Can you work these out from the model? Positions are in its coordinate system, mm. A direction names the side the tool comes from. Coordinates: 2 decimals unless noted, no trailing zeros. Order: outer loops, then holes, each group sorted by start corner. A loop starts at its lowest first (then second) coordinate and runs counter-clockwise, first axis right, second up. Notation, with made-up numbers: (-24, 58) -> (15, 58) arc R32 ccw to (15, 92) -> close; hole circle Ø4 at (54.5, 8.25). An arc over 180 degrees is marked (long way). Answer as CSV lines item,"result".
from build123d import *

# Parameters (mm, degrees)
F0_W     = 101.152622
F0_H     = 124.431356
F1_DEPTH = 2
F2_W     = 101.152622
F2_H     = 124.431356
F2_W_2   = 92.701234
F2_H_2   = 115.979962
F3_DEPTH = 50
F4_W     = 165.897682
F4_H     = 37.940726
F5_DEPTH = 12


with BuildPart() as f1:
    # F0 (on Top) → F1 (new body)
    with BuildSketch(Plane.XY):
        Rectangle(F0_W, F0_H)
    extrude(amount=F1_DEPTH)

    # F2 (on face) → F3 (join)
    with BuildSketch(Plane.XY.offset(2)):
        Rectangle(F2_W, F2_H)
        Rectangle(F2_W_2, F2_H_2, mode=Mode.SUBTRACT)
    extrude(amount=F3_DEPTH)

    # F4 (on Top) → F5 (join)
    with BuildSketch(Plane.XY):
        with Locations((-26.223734, 12.385411)):
            Rectangle(F4_W, F4_H)
    extrude(amount=F5_DEPTH)


solid = f1.part
Q1. Imagine slicing it at C-C (x = -44.5). List the corners of the cut face in (y, z) for me.
Solution:
outline,"(-62.22, 0) -> (62.22, 0) -> (62.22, 52) -> (57.99, 52) -> (57.99, 2) -> (31.36, 2) -> (31.36, 12) -> (-6.58, 12) -> (-6.58, 2) -> (-57.99, 2) -> (-57.99, 52) -> (-62.22, 52) -> close"
Q2. Imagine slicing it at D-D (y = -31.5). List the corners of the cut face in (x, z) for me, and give its area (3 significant figures).
Solution:
outline,"(-50.58, 0) -> (50.58, 0) -> (50.58, 52) -> (46.35, 52) -> (46.35, 2) -> (-46.35, 2) -> (-46.35, 52) -> (-50.58, 52) -> close"
area,"625 mm2"
Q3. Imagine slicing it at B-B (z = 39). List the corners of the cut face in (x, y) for me, and give its area (3 significant figures).
Solution:
outline,"(-50.58, -62.22) -> (50.58, -62.22) -> (50.58, 62.22) -> (-50.58, 62.22) -> close; hole (-46.35, -57.99) -> (46.35, -57.99) -> (46.35, 57.99) -> (-46.35, 57.99) -> close"
area,"1,840 mm2"
Q4. Which directions (+Z, -Z, +X, -X, +Y, -Y) give clear straight access to the entire face, cutting with the end or side of a thin tool? Please do faces 1 (the flat face through (-1, -32, 2)), 2 (the flat face through (54, 13, 12)), 3 (the flat face through (54, 31.356, 6)), 4 (the flat face through (-80, -6.585, 6)).
Solution:
face 1,"+Z"
face 2,"+Z, +X, +Y, -Y"
face 3,"+Z, -Z, +X, +Y"
face 4,"+Z, -Z, -X, -Y"
Q5. If I drill on line 1 (Y direction, x = 15.5, z = 8); line 2 (Y direction, x = 11.5, z = 23.5); line 3 (X direction, y = -31, z = 29.5), over which ranges is the centre line in solid material (lowest first)?
Solution:
line 1,"-62.22 to -57.99, -6.58 to 31.36, 57.99 to 62.22"
line 2,"-62.22 to -57.99, 57.99 to 62.22"
line 3,"-50.58 to -46.35, 46.35 to 50.58"
Q6. We'd pull the mould along X, two halves only. Please class faces 5 (the flat face through (-109.173, 12, 6)), 6 (the flat face through (-80, 13, 12)), 7 (the flat face through (-1, 57.99, 27)): pulls with the +X half, pulls with the -X half, needs draft (parallel to the pull), parting line crosses it, or undercut.
Solution:
face 5,"pulls with the -X half"
face 6,"needs draft"
face 7,"undercut"
Q7. For P1, Ø13.5, axis at x = -2, y = 38.5, coming from the +Z side; P2, Ø9.5, axis at x = -77.5, z = 6, coming from the -Y side; P3, Ø4, axis at y = -34.5, z = 26, coming from the +X side, each with a flat end and sliding along its axis, tell me the tip position at first contact or that it passes through.
Solution:
P1,"z = 2"
P2,"y = -6.58"
P3,"x = 50.58"
Q8. Imagine slicing it at A-A (z = 9). List the corners of the cut face in (x, y) for me, and give its area (3 significant figures).
Solution:
outline,"(-109.17, -6.58) -> (-50.58, -6.58) -> (-50.58, -62.22) -> (50.58, -62.22) -> (50.58, -6.58) -> (56.73, -6.58) -> (56.73, 31.36) -> (50.58, 31.36) -> (50.58, 62.22) -> (-50.58, 62.22) -> (-50.58, 31.36) -> (-109.17, 31.36) -> close; hole (-46.35, -57.99) -> (46.35, -57.99) -> (46.35, -6.58) -> (-46.35, -6.58) -> close; hole (-46.35, 31.36) -> (46.35, 31.36) -> (46.35, 57.99) -> (-46.35, 57.99) -> close"
area,"7,810 mm2"
